Geometry: final body of the model. Coordinates: model frame, mm. Coordinates: 2 decimals unless noted, no trailing zeros. Write each loop counter-clockwise with the first axis right and the second up, starting at its lowest first coordinate (ties: lowest second). Pieces come first, ordered by that corner, then holes. Notation, with made-up numbers: M 88.25,32.5 L 99.25,32.5 A23 cw 99.25,69.5 Z; hole C 35,48 d9. An arc over 180 degrees is marked long. Write item = value, one per line. Start each with the question number.
Item 1: Section C-C on y = 9. Output: boundary loops of the cut face in (x, z), plus the area to 3 significant figures.
Item 2: Pull-direction query (Z, two-part tool) for faces 1 (the flat face through (-4.9, 0, -9.4)), 2 (the flat face through (-5, 15, -10)), 3 (the cylindrical face through (-5.694, 15.196, -1.876)); classes: +Z half, -Z half, draft (parallel to the pull), parting line (faces both ways), or undercut.
Item 3: Section A-A on z = -5. Output: boundary loops of the cut face in (x, y), plus the area to 3 significant figures.
Item 4: Ray query, L1, parallel to X at y = 13.25, z = -5; L2, parallel to X at y = 19.75, z = -6.5. Return the intervals inside material, ascending. Write a range as [from, to].
Item 5: Section B-B on x = -5. Output: boundary loops of the cut face in (y, z).
Autodesk Inventor part; units mm, degrees
ref_plane "YZ Plane" through (0, 0, 0) normal (1, 0, 0) x (0, 1, 0)
ref_plane "XZ Plane" through (0, 0, 0) normal (0, 1, 0) x (-1, 0, 0)
ref_plane "XY Plane" through (0, 0, 0) normal (0, 0, 1) x (1, 0, 0)
sketch "Sketch1" plane through (0, 0, 0) normal (0, 1, 0) x (-1, 0, 0)
  line L0 (0, 0) -> (10, 0)
  line L1 (10, 0) -> (10, -10)
  line L2 (10, -10) -> (0, -10)
  line L3 (0, -10) -> (0, 0)
  dimension "d0" = 10
  dimension "d1" = 10
extrude "Extrusion1" add sketch "Sketch1" along normal blind 30
fillet "Fillet1" radius 2 4 edges at (0, 15, 0) (0, 15, -10) (-10, 15, 0) (-10, 15, -10)
sketch "Sketch2" plane through (0, 30, 0) normal (0, 1, 0) x (1, 0, 0)
  circle A0 centre (-5, 5) radius 3.2
  line L0 (-8, 0) -> (-2, 0)
  line L1 (-10, 8) -> (-10, 2)
  point P0 (0, 0)
  dimension "d5" = 6.4
  dimension "d6" = 5
  dimension "d7" = 5
extrude "Extrusion2" cut sketch "Sketch2" against normal through all
fillet "Fillet2" radius 1 2 edges at (-8.2, 30, -5) (-8.2, 0, -5)
properties part number "30mm_HeatInsertSpacer"
Responses:
q1.outline = M -10,-8 A2 ccw -8,-10 L -2,-10 A2 ccw 0,-8 L 0,-2 A2 ccw -2,0 L -8,0 A2 ccw -10,-2 Z; hole C -5,-5 d6.4
q1.area = 64.4 mm²
q2.face_1 = draft
q2.face_2 = -Z half
q2.face_3 = undercut
q3.outline = M -10,0 L -9.2,0 A1 ccw -8.2,1 L -8.2,29 A1 ccw -9.2,30 L -10,30 Z; M -1.8,1 A1 ccw -0.8,0 L 0,0 L 0,30 L -0.8,30 A1 ccw -1.8,29 Z
q3.area = 107 mm²
q4.L1 = [-10, -8.2], [-1.8, 0]
q4.L2 = [-10, -7.83], [-2.17, 0]
q5.outline = M 0,-10 L 30,-10 L 30,-9.2 A1 ccw 29,-8.2 L 1,-8.2 A1 ccw 0,-9.2 Z; M 0,-0.8 A1 ccw 1,-1.8 L 29,-1.8 A1 ccw 30,-0.8 L 30,0 L 0,0 Z
